Autodesk Inventor part; units mm, degrees
ref_plane "YZ Plane" through (0, 0, 0) normal (1, 0, 0) x (0, 1, 0)
ref_plane "XZ Plane" through (0, 0, 0) normal (0, 1, 0) x (-1, 0, 0)
ref_plane "XY Plane" through (0, 0, 0) normal (0, 0, 1) x (1, 0, 0)
sketch "Sketch1" plane through (0, 0, 0) normal (0, 0, 1) x (1, 0, 0)
  line L0 (0, 0) -> (60, 0)
  line L1 (60, 0) -> (60, 153)
  line L2 (60, 153) -> (0, 153)
  line L3 (0, 153) -> (0, 0)
  dimension "d0" = 153
  dimension "d1" = 60
extrude "Plate1" add sketch "Sketch1" along normal blind 2
sketch "Sketch2" plane through (60, -2, 4) normal (0, -1, 0) x (1, 0, 0)
  line L0 (-60, 0) -> (0, 0)
  line L1 (0, 0) -> (0, 33)
  line L2 (0, 33) -> (-60, 33)
  line L3 (-60, 33) -> (-60, 0)
edge flange "Flange1" height 35 angle 90 thickness 2 bend radius 2 thickness toward (0, -1, 0) relief tear relief width 2 relief depth 1 corner gap 2 corner form 0 edges at (30, 0, 2) (30, 153, 2) wall of the first edge with corners at (0, -2, 4) (60, -2, 4) (60, -2, 37) (0, -2, 37)
bend "Bend1"
corner "Corner1"
sketch "Sketch3" plane through (0, -4, 37) normal (0, -1, 0) x (1, 0, 0)
  line L0 (0, -33) -> (60, -33)
  line L1 (0, -33) -> (0, 0)
  circle A0 centre (15, -22.75) radius 5.25
  point P0 (0, -37)
  dimension "d13" = 15
  dimension "d14" = 10.5
  dimension "d16" = 10.25
extrude "Extrusion1" cut sketch "Sketch3" against normal through all
sketch "Sketch4" plane through (0, 0, 2) normal (0, 0, 1) x (1, 0, 0)
  line L0 (0, 0) -> (0, 153)
  line L1 (60, 153) -> (60, 0)
  circle A0 centre (50, 136.5) radius 2.5
  circle A1 centre (40, 136.5) radius 2.5
  line L2 (60, 76.5) -> (0, 76.5) construction
  circle A2 centre (50, 16.5) radius 2.5
  circle A3 centre (40, 16.5) radius 2.5
  dimension "d20" = 10
  dimension "d21" = 20
  dimension "d22" = 5
  dimension "d23" = 5
  dimension "d24" = 120
extrude "Extrusion2" cut sketch "Sketch4" against normal through all
equation "\"d3\" = BendReliefWidth"
equation "\"d4\" = BendReliefDepth"
equation "\"d5\" = MinimumRemnant"
equation "\"d6\" = BendRadius"
equation "\"d9\" = BendRadius"
equation "\"d10\" = CornerReliefSize"
equation "\"d11\" = GapSize"
equation "\"d12\" = JacobiRadiusSize"
equation "\"BendRadius\" = Thickness"
equation "\"BendReliefWidth\" = Thickness"
equation "\"BendReliefDepth\" = 0.5 * Thickness"
equation "\"CornerReliefSize\" = 4 * Thickness"
equation "\"MinimumRemnant\" = 2 * Thickness"
equation "\"TransitionRadius\" = BendRadius"
equation "\"JacobiRadiusSize\" = BendRadius"
equation "\"GapSize\" = Thickness"
equation "\"d2\" = BendRadius"
properties part number "MotorPlatta"
Could you check a few things on this model? Use its own coordinates, in mm. A direction names the side the tool comes from. Round coordinates to 2 decimals unless told otherwise and drop trailing zeros. Loops run counter-clockwise (first coordinate to the right, second up) from the corner with the lowest first, then second, coordinate; pieces in that order, holes last. Notation, with made-up numbers: M 73,-32.75 L 86,-32.75 A15 cw 86,-22.75 Z; hole C 52,80 d9. An arc over 180 degrees is marked long. Write item = value, one per line.
1. Will this pin go through, and if not, where does the flat tip stop? P1, Ø10, axis at x = 13, y = 15, coming from the -Z side.
Results below:
P1 = 0
2. Thinking about a two-plate mould opening in Z: for faces 1 (the face through (30, -2, 20)), 2 (the face through (11.13, 155.99, 17.8)), 3 (the face through (29.58, 155.859, 1.203)), which applies, +Z half, -Z half, draft (parallel to the pull), parting line (faces both ways), or undercut?
Results below:
face_1 = draft
face_2 = undercut
face_3 = -Z half
3. I want a section at B-B, the plane y = 136.5. Write out the boundary of the cut face in (x, z).
Results below:
outline = M 0,0 L 37.5,0 L 37.5,2 L 0,2 Z; M 42.5,0 L 47.5,0 L 47.5,2 L 42.5,2 Z; M 52.5,0 L 60,0 L 60,2 L 52.5,2 Z
4. I want a section at D-D, the plane z = 34.5. Write out the boundary of the cut face in (x, y).
Results below:
outline = M 0,-4 L 60,-4 L 60,-2 L 0,-2 Z; M 0,155 L 60,155 L 60,157 L 0,157 Z
5. Which directions (+Z, -Z, +X, -X, +Y, -Y) give clear straight access to the entire face, cutting with the end or side of a thin tool? Please do faces 4 (the face through (30, 157, 21)), 5 (the face through (30, 155, 20)).
Results below:
face_4 = +Z, -Z, +X, -X, +Y
face_5 = +Z, +X, -X
6. I want a section at A-A, the plane z = 14.25. Write out the boundary of the cut face in (x, y).
Results below:
outline = M 0,-4 L 9.75,-4 L 9.75,-2 L 0,-2 Z; M 0,155 L 9.75,155 L 9.75,157 L 0,157 Z; M 20.25,-4 L 60,-4 L 60,-2 L 20.25,-2 Z; M 20.25,155 L 60,155 L 60,157 L 20.25,157 Z
7. I want a section at C-C, the plane x = 50. Write out the boundary of the cut face in (y, z), and give its area (3 significant figures).
Results below:
outline = M -4,4 A4 ccw 0,0 L 14,0 L 14,2 L 0,2 A2 cw -2,4 L -2,37 L -4,37 Z; M 19,0 L 134,0 L 134,2 L 19,2 Z; M 139,0 L 153,0 A4 ccw 157,4 L 157,37 L 155,37 L 155,4 A2 cw 153,2 L 139,2 Z
area = 437 mm²
8. I need wall thicknesses on probe 1 along X at (y, z) = (136.5, 0.7); probe 2 along Y at (x, z) = (16, 33); probe 3 along X at (y, z) = (156, 14). Which ranges of each line are inside material? Lowest first, please.
Results below:
probe_1 = 0 to 37.5, 42.5 to 47.5, 52.5 to 60
probe_2 = -4 to -2, 155 to 157
probe_3 = 0 to 9.76, 20.24 to 60
